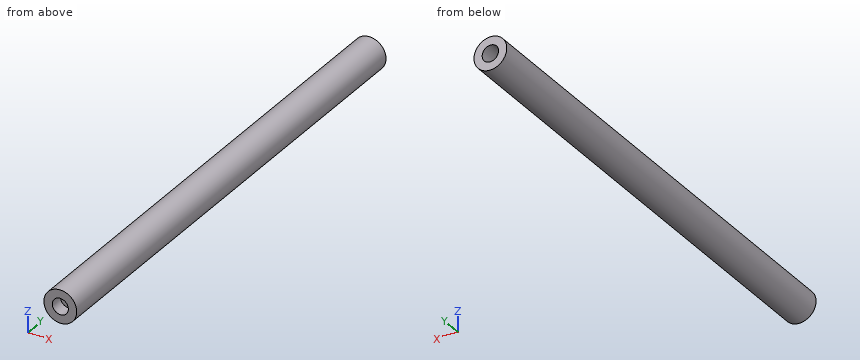
Autodesk Fusion 360 part; units mm, degrees
sketch "Sketch1" plane through (0, 0, 0) normal (0, 1, 0) x (1, 0, 0)
sketch "Sketch2" plane through (0, 0, 0) normal (0, 1, 0) x (1, 0, 0)
  circle A0 centre (0, 0) radius 5
  dimension "d21" = 10
extrude "Extrude3" add sketch "Sketch2" along normal blind 150
hole "Hole6" at (0, 150, 0) direction (0, -1, 0) diameter 5 depth 50 tip angle 180
hole "Hole7" at (0, 0, 0) direction (0, 1, 0) diameter 4.9 depth 4 tip angle 180
The model under review builds one solid part; all positions refer to its coordinate system, in mm. Coordinates: 2 decimals unless noted, no trailing zeros. Loops run counter-clockwise (first coordinate to the right, second up) from the corner with the lowest first, then second, coordinate; pieces in that order, holes last. Notation, with made-up numbers: (49, -18.5) -> (104, -18.5) arc R20 ccw to (104, 13.5) -> close; hole circle Ø7 at (55.5, 26). An arc over 180 degrees is marked (long way). Use a Markdown table: item, result. Add a question column.
1. Add section D-D on y = 79. Write out the cut boundary in (x, z), plus the area to 3 significant figures.
2. Add section A-A on x = 0. Write out the cut boundary in (y, z).
3. Add section B-B on z = 0. Write out the cut boundary in (x, y).
4. Clearance check with flat-ended pins moving along their axes: pin 1 Ø1.5 at (y, z) = (89, 1) entering from +X; pin 2 Ø6 at (y, z) = (99, 4) entering from +X; pin 3 Ø5 at (y, z) = (124.5, 4) entering from +X. State where each tip first meets the part, or that it passes through.
5. To check wall thickness, follow line 1 (X direction, y = 126.5, z = 0); line 2 (X direction, y = 13, z = 0.25). State the ranges of each line that lie inside material, in increasing order.
6. Add section C-C on y = 114. Write out the cut boundary in (x, z).
Returned:
| question | item | result |
|---|---|---|
| 1 | outline | circle Ø10 at (0, 0) |
| 1 | area | 78.5 mm² |
| 2 | outline | (0, -5) -> (150, -5) -> (150, -2.5) -> (100, -2.5) -> (100, 2.5) -> (150, 2.5) -> (150, 5) -> (0, 5) -> (0, 2.45) -> (4, 2.45) -> (4, -2.45) -> (0, -2.45) -> close |
| 3 | outline | (-5, 0) -> (-2.45, 0) -> (-2.45, 4) -> (2.45, 4) -> (2.45, 0) -> (5, 0) -> (5, 150) -> (2.5, 150) -> (2.5, 100) -> (-2.5, 100) -> (-2.5, 150) -> (-5, 150) -> close |
| 4 | pin 1 | stops at x = 4.99 |
| 4 | pin 2 | stops at x = 4.9 |
| 4 | pin 3 | stops at x = 4.77 |
| 5 | line 1 | x = -5 to -2.5, 2.5 to 5 |
| 5 | line 2 | x = -4.99 to 4.99 |
| 6 | outline | circle Ø10 at (0, 0); hole circle Ø5 at (0, 0) |
